Autodesk Inventor part; units mm, degrees
ref_plane "YZ Plane" through (0, 0, 0) normal (1, 0, 0) x (0, 1, 0)
ref_plane "XZ Plane" through (0, 0, 0) normal (0, 1, 0) x (-1, 0, 0)
ref_plane "XY Plane" through (0, 0, 0) normal (0, 0, 1) x (1, 0, 0)
sketch "Esquisse1" plane through (0, 0, 0) normal (0, 1, 0) x (-1, 0, 0)
  line L0 (3, -3) -> (-3, -3)
  line L1 (-3, -3) -> (-3, 3)
  line L2 (-3, 3) -> (3, 3)
  line L3 (3, 3) -> (3, -3)
  point P0 (0, 0)
  dimension "d0" = 3
  dimension "d1" = 6
  dimension "d2" = 6
  dimension "d3" = 3
extrude "Extrusion1" add sketch "Esquisse1" along normal blind 4
sketch "Esquisse2" plane through (0, 4, 0) normal (0, 1, 0) x (1, 0, 0)
  circle A0 centre (0, 0) radius 1.75
  dimension "d6" = 3.5
extrude "Extrusion2" add sketch "Esquisse2" along normal blind 1.5
sketch "Esquisse3" plane through (0, 4, 0) normal (0, 1, 0) x (1, 0, 0)
  circle A0 centre (-2.2, -2.2) radius 0.6
  line L0 (-3, -3) -> (3, -3)
  line L1 (-3, 3) -> (-3, -3)
  circle A1 centre (2.2, -2.2) radius 0.6
  circle A2 centre (-2.2, 2.2) radius 0.6
  circle A3 centre (2.2, 2.2) radius 0.6
  point P0 (0, 0)
  dimension "d9" = 0.8
  dimension "d10" = 0.8
  dimension "d11" = 1.2
  dimension "d14" = 4.4
  dimension "d17" = 4.4
extrude "Extrusion3" add sketch "Esquisse3" along normal blind 0.4
sketch "Esquisse4" plane through (0, 0, 0) normal (0, -1, 0) x (1, 0, 0)
  line L0 (-3, 3) -> (3, 3)
  line L1 (2.4, 3) -> (1.6, 3)
  line L2 (1.6, 3) -> (1.6, 5)
  line L3 (1.6, 5) -> (2.4, 5)
  line L4 (2.4, 5) -> (2.4, 3)
  line L5 (3, -3) -> (3, 3)
  line L6 (2.4, -5) -> (1.6, -5)
  line L7 (1.6, -5) -> (1.6, -3)
  line L8 (1.6, -3) -> (2.4, -3)
  line L9 (2.4, -3) -> (2.4, -5)
  line L10 (-1.6, 3) -> (-2.4, 3)
  line L11 (-2.4, 3) -> (-2.4, 5)
  line L12 (-2.4, 5) -> (-1.6, 5)
  line L13 (-1.6, 5) -> (-1.6, 3)
  line L14 (-1.6, -5) -> (-2.4, -5)
  line L15 (-2.4, -5) -> (-2.4, -3)
  line L16 (-2.4, -3) -> (-1.6, -3)
  line L17 (-1.6, -3) -> (-1.6, -5)
  point P0 (0, 0)
  dimension "d22" = 2
  dimension "d23" = 0.8
  dimension "d24" = 0.6
  dimension "d27" = 8
  dimension "d30" = 4
extrude "Extrusion4" add sketch "Esquisse4" against normal blind 0.5
fillet "Congé1" radius 0.5 4 edges at (1.6, 4.4, 2.2) (-2.8, 4.4, 2.2) (-2.8, 4.4, -2.2) (1.6, 4.4, -2.2)
fillet "Congé2" radius 0.1 1 edges at (-1.75, 5.5, 0)
fillet "Congé3" radius 0.1 4 edges at (3, 2, 3) (3, 2, -3) (-3, 2, -3) (-3, 2, 3)
equation "\"d10\" = d9"
properties part number "Touch Button"
Geometry: final body of the model. Coordinates: model frame, mm. A direction names the side the tool comes from. Give positions to 0.01 mm unless a question says otherwise; leave off trailing zeros. Write each loop counter-clockwise with the first axis right and the second up, starting at its lowest first coordinate (ties: lowest second). Pieces come first, ordered by that corner, then holes.
1. Section query A-A, the plane z = -3.5. Return loops of the section in (x, y), then the cut area to 3 significant figures.
2. Section query B-B, the plane y = 3.25. Return loops of the section in (x, z), then the cut area to 3 significant figures.
3. Section query C-C, the plane x = 0. Return loops of the section in (y, z), then the cut area to 3 significant figures.
4. Draft query along Z for faces 1 (the flat face through (-1.3, 4, 1.4)), 2 (the flat face through (-3, 2, 0)). Return one class per face: released by +Z, released by -Z, zero draft, split by the parting line, or undercut.
5. Section query D-D, the plane z = 0. Return loops of the section in (x, y), then the cut area to 3 significant figures.
6. Line query: probe 1 along Z at (x, y) = (-1.5, 1.95); probe 2 along Y at (x, z) = (1.25, -1.5); probe 3 along Z at (x, y) = (2.4, 4.1). Output: solid intervals per line, ascending.
7. Reachability of faces 3 (the flat face through (2, 0.5, 4)), 4 (the cylindrical face through (1.617, 4.69, -0.67)), 5 (the flat face through (0, 0, 0)) from +Z, -Z, +X, -X, +Y, -Y: full face, straight path, thin tool, end or side. Return the list, or none.
8. Pin query (flat end, axial travel): P1, Ø0.9, axis at x = 2, z = 4, coming from the +Y side; P2, Ø2, axis at x = 0, y = 2.5, coming from the +Z side; P3, Ø0.6, axis at y = 0.5, z = 4.5, coming from the +X side. Return the tip coordinate at first contact, or that it passes through.
Computed:
1. outline: (-2.4, 0) - (-1.6, 0) - (-1.6, 0.5) - (-2.4, 0.5) - close; (1.6, 0) - (2.4, 0) - (2.4, 0.5) - (1.6, 0.5) - close
1. area: 0.800 mm2
2. outline: (-3, -2.9) arc R0.1 ccw to (-2.9, -3) - (2.9, -3) arc R0.1 ccw to (3, -2.9) - (3, 2.9) arc R0.1 ccw to (2.9, 3) - (-2.9, 3) arc R0.1 ccw to (-3, 2.9) - close
2. area: 36.0 mm2
3. outline: (0, -3) - (4, -3) - (4, -1.75) - (5.4, -1.75) arc R0.1 ccw to (5.5, -1.65) - (5.5, 1.65) arc R0.1 ccw to (5.4, 1.75) - (4, 1.75) - (4, 3) - (0, 3) - close
3. area: 29.2 mm2
4. face 1: undercut
4. face 2: zero draft
5. outline: (-3, 0) - (3, 0) - (3, 4) - (1.75, 4) - (1.75, 5.4) arc R0.1 ccw to (1.65, 5.5) - (-1.65, 5.5) arc R0.1 ccw to (-1.75, 5.4) - (-1.75, 4) - (-3, 4) - close
5. area: 29.2 mm2
6. probe 1: z = -3 to 3
6. probe 2: y = 0 to 4
6. probe 3: z = -2.73 to -1.67, 1.67 to 2.73
7. face 3: +Z, +X, -X, +Y
7. face 4: +Y
7. face 5: +Z, -Z, +X, -X, -Y
8. P1: stops at y = 0.5
8. P2: stops at z = 3
8. P3: stops at x = 2.4
